```python
from build123d import *

# Parameters (mm, degrees)
SKETCH_1_R          = 10.25
EXTRUDE_1_DEPTH     = 2
SKETCH_2_R          = 4
SKETCH_2_R_2        = 3
EXTRUDE_2_DEPTH     = 3
SKETCH_4_R          = 1
CUT_EXTRUDE_1_DEPTH = 3


with BuildPart() as part:
    # 草图1 → 凸台-拉伸1 (new body)
    with BuildSketch(Plane(origin=(0, 0, 0), x_dir=(1, 0, 0), z_dir=(0, 1, 0))):
        Circle(SKETCH_1_R)
    extrude(amount=EXTRUDE_1_DEPTH)

    # 草图2 → 凸台-拉伸2 (add)
    with BuildSketch(Plane.XZ):
        Circle(SKETCH_2_R)
        Circle(SKETCH_2_R_2, mode=Mode.SUBTRACT)
    extrude(amount=EXTRUDE_2_DEPTH)

    # 草图4 → 切除-拉伸1 (cut)
    with BuildSketch(Plane(origin=(0, 2, 0), x_dir=(1, 0, 0), z_dir=(0, 1, 0))):
        with Locations((-7, 0)):
            Circle(SKETCH_4_R)
        with Locations((0, 7)):
            Circle(SKETCH_4_R)
        with Locations((7, 0)):
            Circle(SKETCH_4_R)
        with Locations((0, -7)):
            Circle(SKETCH_4_R)
    extrude(amount=-CUT_EXTRUDE_1_DEPTH, mode=Mode.SUBTRACT)


solid = part.part
```
Geometry check sheet. Reference: the model listing, model coordinates, mm. A direction names the side the tool comes from. Coordinates: 2 decimals unless noted, no trailing zeros. Write each loop counter-clockwise with the first axis right and the second up, starting at its lowest first coordinate (ties: lowest second). Pieces come first, ordered by that corner, then holes. Notation, with made-up numbers: M 87.5,-38.75 L 125.5,-38.75 A20 ccw 125.5,-3.75 Z; hole C -11.75,54 d8. An arc over 180 degrees is marked long. Use one line per item in the form item = value. Start each with the question number.
1) Section check C-C on y = -1.7. Enter the section's corners in (x, z), and give its area (3 significant figures).
2) Go/stop test with flat-tipped pins: pin 1 Ø1.8 at (x, z) = (0, 7) entering from -Y; pin 2 Ø5 at (x, z) = (1, 4.5) entering from -Y; pin 3 Ø1.8 at (x, z) = (-0.5, -1.5) entering from -Y. Record where each tip stops, or that it passes through.
3) Section check A-A on x = 0. Enter the section's corners in (y, z), and give its area (3 significant figures).
4) Release check for a two-part mould opening along Z. For faces 1 (the cylindrical face through (-2.222, 0.986, 10.006)), 2 (the flat face through (1, -3, 3)), 3 (the cylindrical face through (0, 1, 6)), 4 (the cylindrical face through (0, 1, -8)) record: pulls with the +Z half, pulls with the -Z half, needs draft (parallel to the pull), parting line crosses it, or undercut.
5) Section check D-D on x = -7. Enter the section's corners in (y, z), and give its area (4 significant figures).
6) Section check B-B on z = 0. Enter the section's corners in (x, y), and give its area (3 significant figures).
7) Set-up check for faces 5 (the cylindrical face through (-7.8, 1, 0.6)), 6 (the flat face through (-0.1, 0, 4.4)): record each of +Z, -Z, +X, -X, +Y, -Y from which the full face is reachable in a straight line by a thin tool's end or side.
8) Thickness scan on probe 1 along Z at (x, y) = (0, 0.7); probe 2 along Y at (x, z) = (1.75, -2.25). Record the ranges inside material, lowest first. Write a range as from..to.
Responses:
q1.outline = C 0,0 d8; hole C 0,0 d6
q1.area = 22.0 mm2
q2.pin_1 = through
q2.pin_2 = -3
q2.pin_3 = 0
q3.outline = M -3,-4 L 0,-4 L 0,-6 L 2,-6 L 2,6 L 0,6 L 0,4 L -3,4 L -3,3 L 0,3 L 0,-3 L -3,-3 Z; M 0,-10.25 L 2,-10.25 L 2,-8 L 0,-8 Z; M 0,8 L 2,8 L 2,10.25 L 0,10.25 Z
q3.area = 39.0 mm2
q4.face_1 = parting line crosses it
q4.face_2 = needs draft
q4.face_3 = undercut
q4.face_4 = undercut
q5.outline = M 0,-7.49 L 2,-7.49 L 2,-1 L 0,-1 Z; M 0,1 L 2,1 L 2,7.49 L 0,7.49 Z
q5.area = 25.95 mm2
q6.outline = M -10.25,0 L -8,0 L -8,2 L -10.25,2 Z; M -6,0 L -4,0 L -4,-3 L -3,-3 L -3,0 L 3,0 L 3,-3 L 4,-3 L 4,0 L 6,0 L 6,2 L -6,2 Z; M 8,0 L 10.25,0 L 10.25,2 L 8,2 Z
q6.area = 39.0 mm2
q7.face_5 = +Y, -Y
q7.face_6 = -Y
q8.probe_1 = -10.25..-8, -6..6, 8..10.25
q8.probe_2 = 0..2
